Read the model definition and answer for the solid it produces. Units are mm, in the model's axes. Face numbers are marked on the shaded views. A direction names the side the tool comes from. Coordinates: 2 decimals unless noted, no trailing zeros. Write each loop counter-clockwise with the first axis right and the second up, starting at its lowest first coordinate (ties: lowest second). Pieces come first, ordered by that corner, then holes. Notation, with made-up numbers: (9, 72.25) - (32, 72.25) arc R30 ccw to (32, 108.25) - close; hole circle Ø7 at (68.5, -25). An arc over 180 degrees is marked (long way). Return JSON: item names as keys, results as strings.
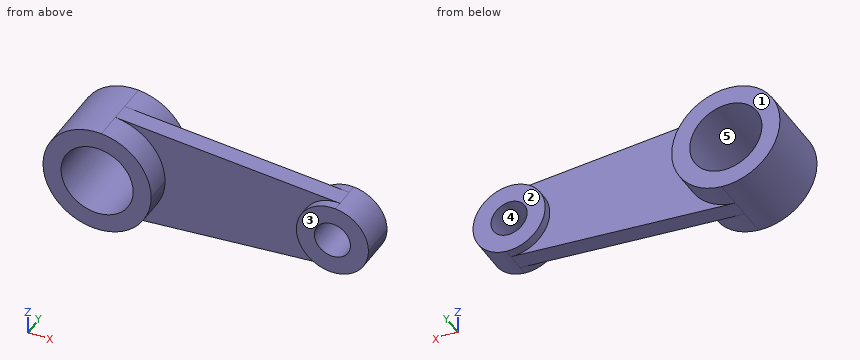
```python
from build123d import *

# Parameters (mm, degrees)
F1_DEPTH = 10
F0_R     = 20
F2_DEPTH = 25
F3_DEPTH = 15
F0_R_2   = 10
F4_DEPTH = 15
F5_DEPTH = 5


with BuildPart() as f1:
    # F0 (on Front) → F1 (new body)
    with BuildSketch(Plane.XZ):
        with BuildLine():
            ThreePointArc((-77.264525, 29.904412), (-57.614458, 20.349593), (-49.657463, 0))
            ThreePointArc((-49.657463, 0), (-57.614458, -20.349593), (-77.264525, -29.904412))
            Line((-77.264525, -29.904412), (47.306721, -19.936275))
            ThreePointArc((47.306721, -19.936275), (25.711429, 0), (47.306721, 19.936275))
            Line((47.306721, 19.936275), (-77.264525, 29.904412))
        make_face()
    extrude(amount=F1_DEPTH)

    # F0 (on Front) → F2 (join)
    with BuildSketch(Plane.XZ):
        with BuildLine():
            ThreePointArc((-77.264525, -29.904412), (-57.614458, -20.349593), (-49.657463, 0))
            ThreePointArc((-49.657463, 0), (-57.614458, 20.349593), (-77.264525, 29.904412))
            ThreePointArc((-77.264525, 29.904412), (-109.657463, 0), (-77.264525, -29.904412))
        make_face()
        with Locations((-79.657463, 0)):
            Circle(F0_R, mode=Mode.SUBTRACT)
    extrude(amount=F2_DEPTH)

    # F0 (on Front) → F3 (join)
    with BuildSketch(Plane.XZ):
        with BuildLine():
            ThreePointArc((-77.264525, -29.904412), (-57.614458, -20.349593), (-49.657463, 0))
            ThreePointArc((-49.657463, 0), (-57.614458, 20.349593), (-77.264525, 29.904412))
            ThreePointArc((-77.264525, 29.904412), (-109.657463, 0), (-77.264525, -29.904412))
        make_face()
        with Locations((-79.657463, 0)):
            Circle(F0_R, mode=Mode.SUBTRACT)
    extrude(amount=-F3_DEPTH)

    # F0 (on Front) → F4 (join)
    with BuildSketch(Plane.XZ):
        with BuildLine():
            ThreePointArc((65.711429, 0), (60.406766, 13.566395), (47.306721, 19.936275))
            ThreePointArc((47.306721, 19.936275), (25.711429, 0), (47.306721, -19.936275))
            ThreePointArc((47.306721, -19.936275), (60.406766, -13.566395), (65.711429, 0))
        make_face()
        with Locations((45.711429, 0)):
            Circle(F0_R_2, mode=Mode.SUBTRACT)
    extrude(amount=F4_DEPTH)

    # F0 (on Front) → F5 (join)
    with BuildSketch(Plane.XZ):
        with BuildLine():
            ThreePointArc((65.711429, 0), (60.406766, 13.566395), (47.306721, 19.936275))
            ThreePointArc((47.306721, 19.936275), (25.711429, 0), (47.306721, -19.936275))
            ThreePointArc((47.306721, -19.936275), (60.406766, -13.566395), (65.711429, 0))
        make_face()
        with Locations((45.711429, 0)):
            Circle(F0_R_2, mode=Mode.SUBTRACT)
    extrude(amount=-F5_DEPTH)


solid = f1.part
```
(1) A cutting plane is placed at C-C (z = 13). Determine the outline of the cut face in (x, y), and give its area (3 significant figures).
Answer:
{"outline": "(-106.69, -25) - (-94.86, -25) - (-94.86, 15) - (-106.69, 15) - close; (-64.46, -25) - (-52.62, -25) - (-52.62, -10) - (30.51, -10) - (30.51, -15) - (60.91, -15) - (60.91, 5) - (30.51, 5) - (30.51, 0) - (-52.62, 0) - (-52.62, 15) - (-64.46, 15) - close", "area": "2,390 mm²"}
(2) A cutting plane is placed at A-A (y = -13). Determine the outline of the cut face in (x, z).
Answer:
{"outline": "circle Ø60 at (-79.66, 0); (47.31, -19.94) arc R20 ccw to (47.31, 19.94) arc R20 ccw (long way) to start; hole circle Ø40 at (-79.66, 0); hole circle Ø20 at (45.71, 0)"}
(3) Determine the mould class of the marked faces 3, 4 and 5 for opening direction Z: +Z half, -Z half, draft (parallel to the pull), parting line (faces both ways), or undercut.
Answer:
{"face 3": "draft", "face 4": "undercut", "face 5": "undercut"}
(4) Which of the six approach directions +Z, -Z, +X, -X, +Y, -Y give full straight-line access (tool end or side, diameter ignored) to the marked faces 1 and 2?
Answer:
{"face 1": "+Z, -Z, +X, -X, +Y", "face 2": "+Z, -Z, +X, +Y"}
(5) Flat-ended cylindrical pins translate along their axes: P1, Ø12, axis at y = -8, z = 14, coming from the -X side; P2, Ø3, axis at x = -13, z = 15.5, coming from the -Y side; P3, Ø8, axis at y = 4.5, z = 8.5, coming from the -X side. Find the tip coordinate at first contact, or state that the pin passes through.
Answer:
{"P1": "x = -108.57", "P2": "y = -10", "P3": "x = -109.32"}
(6) Straight lines are drawn through the part: line 1 (X direction, y = -5, z = -8.5); line 2 (Y direction, x = -32.5, z = -13.5); line 3 (X direction, y = 7, z = -18.5). For each, find the intervals that lie inside material, in ascending order. Write a range as from..to.
Answer:
{"line 1": "-108.43..-97.76, -61.55..40.44, 50.98..63.82", "line 2": "-10..0", "line 3": "-103.27..-87.26, -72.06..-56.04"}
(7) A cutting plane is placed at B-B (y = -5). Determine the outline of the cut face in (x, z).
Answer:
{"outline": "(-77.26, -29.9) - (47.31, -19.94) arc R20 ccw to (47.31, 19.94) - (-77.26, 29.9) arc R30 ccw (long way) to start; hole circle Ø40 at (-79.66, 0); hole circle Ø20 at (45.71, 0)"}
(8) A cutting plane is placed at D-D (z = -12). Determine the outline of the cut face in (x, y).
Answer:
{"outline": "(-107.15, -25) - (-95.66, -25) - (-95.66, 15) - (-107.15, 15) - close; (-63.66, -25) - (-52.16, -25) - (-52.16, -10) - (29.71, -10) - (29.71, -15) - (61.71, -15) - (61.71, 5) - (29.71, 5) - (29.71, 0) - (-52.16, 0) - (-52.16, 15) - (-63.66, 15) - close"}
